Design review of the part built by this model. Coordinates are the model's own, in mm. Give positions to 0.01 mm unless a question says otherwise; leave off trailing zeros. Order: outer loops, then holes, each group sorted by start corner. A loop starts at its lowest first (then second) coordinate and runs counter-clockwise, first axis right, second up. Notation, with made-up numbers: M 74.5,-33.75 L 95.5,-33.75 A34 ccw 95.5,-2.75 Z; hole C 84,-2 d7. An arc over 180 degrees is marked long. Answer as a JSON object with one key per item and string values.
from build123d import *

# Parameters (mm, degrees)
BOSS_EXTRUDE1_DEPTH = 120
SHELL4_START        = 3
SHELL4_DEPTH        = 114
SKETCH12_W          = 3.498967662
SKETCH12_H          = 114
CUT_EXTRUDE5_DEPTH  = 2
SKETCH9_R           = 1.004458273
BOSS_EXTRUDE5_DEPTH = 10
CUT_EXTRUDE6_DEPTH  = 10
SKETCH14_W          = 1
SKETCH14_H          = 12.98385937
SKETCH14_H_2        = 14.006550136
BOSS_EXTRUDE6_DEPTH = 20


# Read off the part's stored shape, not the designer's step: Shell4
with BuildPart() as part:
    # Sketch1 → Boss-Extrude1 (new body)
    with BuildSketch(Plane(origin=(0, 0, 0), x_dir=(1, 0, 0), z_dir=(0, 1, 0))):
        with BuildLine():
            Line((-74.162924852, 98.042139327), (-73.832168128, 178.220414973))
            Line((-73.832168128, 178.220414973), (-68.833436902, 178.220414973))
            Line((-68.833436902, 178.220414973), (-68.833436902, 98.042139327))
            add(Edge.make_bspline(
                [(-68.833436902, 98.042139327), (-69.18939253, 31.860054141), (-32.378727908, -28.786275828)],
                knots=[0, 0, 0, 1, 1, 1], degree=2))
            Line((-32.378727908, -28.786275828), (-35.878727908, -35.78423441))
            add(Edge.make_bspline(
                [(-74.162924852, 98.042139327), (-75.763847477, 27.752135338), (-35.878727908, -35.78423441)],
                knots=[0, 0, 0, 1, 1, 1], degree=2))
        make_face()
    extrude(amount=BOSS_EXTRUDE1_DEPTH)

    # Shell4 outline → Shell4 (cut)
    with BuildSketch(Plane(origin=(0, 0, 0), x_dir=(1, 0, 0), z_dir=(0, 1, 0)).offset(SHELL4_START)):
        with BuildLine():
            Line((-70.8445184, 175.220414973), (-71.163065765, 98.001792885))
            add(Edge.make_bspline(
                [(-71.163065765, 98.001792885), (-71.16307999, 98.001168327), (-71.163094215, 98.000543769), (-71.16310844, 97.999919211), (-71.163122665, 97.999294653), (-71.16313689, 97.998670095), (-71.163151114, 97.998045537), (-71.163165339, 97.997420979), (-71.163179564, 97.996796421), (-71.163193789, 97.996171862), (-71.163208014, 97.995547304), (-71.163222239, 97.994922746), (-71.163236464, 97.994298188), (-71.163250689, 97.99367363), (-71.163293111, 97.991811054), (-71.163321308, 97.990573036), (-71.163349505, 97.989335018), (-71.163377702, 97.988097001), (-71.163405899, 97.986858982), (-71.163434097, 97.985620965), (-71.163462293, 97.984382945), (-71.163490491, 97.98314493), (-71.163518687, 97.98190691), (-71.163546885, 97.980668893), (-71.163575081, 97.979430874), (-71.163603278, 97.978192857), (-71.163631475, 97.976954838), (-71.163673771, 97.975097811), (-71.16368819, 97.974464701), (-71.163699727, 97.973958392), (-71.163723187, 97.972927066), (-71.163717996, 97.973159219), (-71.163755945, 97.971484687), (-71.163749131, 97.971794066), (-71.163775505, 97.970626161), (-71.163784451, 97.97023953), (-71.163799423, 97.969578445), (-71.163813375, 97.968966514), (-71.163827192, 97.968358956), (-71.163841117, 97.967746949), (-71.163868925, 97.96652446), (-71.163882828, 97.965913216), (-71.163896729, 97.965301972), (-71.163910628, 97.964690728), (-71.163924525, 97.964079485), (-71.163938422, 97.963468242), (-71.163952315, 97.962856999), (-71.163966208, 97.962245757), (-71.163980098, 97.961634515), (-71.163993987, 97.961023273), (-71.164007875, 97.960412031), (-71.16402176, 97.95980079), (-71.164035644, 97.959189549), (-71.164105055, 97.956133346), (-71.164160555, 97.953688388), (-71.16421603, 97.951243436), (-71.164271474, 97.948798484), (-71.164326897, 97.946353546), (-71.164382282, 97.943908598), (-71.164437654, 97.941463673), (-71.164492984, 97.939018734), (-71.164548299, 97.936573815), (-71.164603577, 97.93412889), (-71.164658834, 97.931683976), (-71.16471406, 97.929239064), (-71.16476926, 97.926794157), (-71.164934778, 97.919459451), (-71.165045014, 97.914569665), (-71.165155139, 97.909679898), (-71.165265157, 97.904790149), (-71.165375062, 97.899900419), (-71.165484862, 97.895010708), (-71.165594548, 97.890121015), (-71.165704128, 97.885231341), (-71.165813596, 97.880341685), (-71.165922956, 97.875452049), (-71.166032206, 97.87056243), (-71.166141347, 97.86567283), (-71.166250378, 97.860783249), (-71.166577142, 97.846114561), (-71.166794547, 97.83633551), (-71.167011514, 97.826556534), (-71.167228044, 97.816777632), (-71.167444133, 97.806998804), (-71.167659788, 97.797220051), (-71.167875001, 97.787441372), (-71.16808978, 97.777662768), (-71.168304117, 97.767884237), (-71.168518019, 97.758105782), (-71.168731482, 97.7483274), (-71.168944507, 97.738549093), (-71.169157093, 97.72877086), (-71.170217838, 97.679880069), (-71.171059425, 97.640768626), (-71.171894004, 97.601658372), (-71.172721576, 97.56254931), (-71.173542137, 97.523441433), (-71.174355694, 97.484334754), (-71.175162237, 97.445229255), (-71.175961779, 97.406124956), (-71.176754307, 97.367021836), (-71.177539831, 97.327919914), (-71.178318344, 97.288819177), (-71.179089851, 97.249719631), (-71.179854349, 97.210621274), (-71.183641802, 97.015135438), (-71.186559636, 96.858765798), (-71.189365345, 96.702415187), (-71.192058927, 96.546083598), (-71.194640389, 96.389771034), (-71.197109723, 96.233477481), (-71.199466944, 96.077202952), (-71.201712036, 95.920947426), (-71.203845018, 95.764710916), (-71.205865876, 95.608493406), (-71.207774621, 95.452294903), (-71.20957125, 95.296115396), (-71.211255765, 95.139954887), (-71.215972974, 94.671530339), (-71.21866933, 94.359323281), (-71.220917246, 94.047192171), (-71.222716731, 93.735136985), (-71.224067792, 93.423157694), (-71.224970441, 93.111254278), (-71.225424682, 92.799426705), (-71.22543053, 92.487674957), (-71.224987988, 92.175999001), (-71.224097069, 91.864398817), (-71.222757779, 91.552874376), (-71.220970129, 91.241425656), (-71.218734126, 90.930052628), (-71.210681088, 89.996160551), (-71.203519041, 89.373868515), (-71.194563692, 88.751878946), (-71.183815094, 88.130191631), (-71.171273301, 87.508806354), (-71.156938367, 86.887722903), (-71.140810347, 86.266941062), (-71.122889291, 85.646460617), (-71.103175256, 85.026281355), (-71.081668294, 84.406403059), (-71.058368459, 83.786825518), (-71.033275804, 83.167548515), (-71.006390383, 82.548571838), (-70.920355984, 80.692542137), (-70.855828771, 79.456389412), (-70.784130946, 78.221435319), (-70.70526281, 76.987678074), (-70.619224622, 75.75511588), (-70.52601661, 74.52374694), (-70.425638953, 73.293569436), (-70.318091806, 72.064581558), (-70.20337527, 70.836781468), (-70.081489423, 69.610167339), (-69.952434295, 68.384737319), (-69.816209883, 67.16048956), (-69.672816143, 65.937422197), (-69.221126701, 62.271755688), (-68.891322913, 59.832692682), (-68.532840831, 57.398329004), (-68.145679077, 54.968649529), (-67.729835685, 52.543639338), (-67.285308121, 50.123283736), (-66.812093252, 47.707568223), (-66.310187385, 45.296478532), (-65.779586225, 42.890000586), (-65.220284915, 40.488120539), (-64.632278003, 38.090824743), (-64.015559465, 35.698099773), (-63.370122691, 33.309932408), (-61.444530757, 26.501652756), (-60.094120868, 22.092657129), (-58.644686559, 17.699242409), (-57.096177659, 13.321333259), (-55.448539032, 8.958860031), (-53.701711499, 4.611759301), (-51.855632693, 0.279974273), (-49.910237914, -4.036544954), (-47.865460912, -8.33784126), (-45.721234657, -12.6239505), (-43.477492061, -16.894901644), (-41.134166666, -21.150717052), (-38.691193295, -25.391412877), (-36.148508666, -29.616999611)],
                knots=[-0.000198917, -0.000198917, -0.000198917, -0.000198917, -0.000198917, -0.000198917, -0.000198917, -0.000198917, -0.000198917, -0.000198917, -0.000198917, -0.000198917, -0.000198917, -0.000198917, -0.000198917, -0.000136719, -0.000136719, -0.000136719, -0.000136719, -0.000136719, -0.000136719, -0.000136719, -0.000136719, -0.000136719, -0.000136719, -0.000136719, -0.000136719, -0.000136719, -1.3428e-05, -1.3428e-05, -1.3428e-05, -1.3428e-05, -1.3428e-05, -1.3428e-05, -1.3428e-05, -1.3428e-05, -1.3428e-05, -1.3428e-05, -1.3428e-05, -1.3428e-05, -1.3428e-05, 4.8218e-05, 4.8218e-05, 4.8218e-05, 4.8218e-05, 4.8218e-05, 4.8218e-05, 4.8218e-05, 4.8218e-05, 4.8218e-05, 4.8218e-05, 4.8218e-05, 4.8218e-05, 4.8218e-05, 0.000109863, 0.000109863, 0.000109863, 0.000109863, 0.000109863, 0.000109863, 0.000109863, 0.000109863, 0.000109863, 0.000109863, 0.000109863, 0.000109863, 0.000109863, 0.000356445, 0.000356445, 0.000356445, 0.000356445, 0.000356445, 0.000356445, 0.000356445, 0.000356445, 0.000356445, 0.000356445, 0.000356445, 0.000356445, 0.000356445, 0.000849609, 0.000849609, 0.000849609, 0.000849609, 0.000849609, 0.000849609, 0.000849609, 0.000849609, 0.000849609, 0.000849609, 0.000849609, 0.000849609, 0.000849609, 0.001835937, 0.001835937, 0.001835937, 0.001835937, 0.001835937, 0.001835937, 0.001835937, 0.001835937, 0.001835937, 0.001835937, 0.001835937, 0.001835937, 0.001835937, 0.00578125, 0.00578125, 0.00578125, 0.00578125, 0.00578125, 0.00578125, 0.00578125, 0.00578125, 0.00578125, 0.00578125, 0.00578125, 0.00578125, 0.00578125, 0.0215625, 0.0215625, 0.0215625, 0.0215625, 0.0215625, 0.0215625, 0.0215625, 0.0215625, 0.0215625, 0.0215625, 0.0215625, 0.0215625, 0.0215625, 0.053125, 0.053125, 0.053125, 0.053125, 0.053125, 0.053125, 0.053125, 0.053125, 0.053125, 0.053125, 0.053125, 0.053125, 0.053125, 0.11625, 0.11625, 0.11625, 0.11625, 0.11625, 0.11625, 0.11625, 0.11625, 0.11625, 0.11625, 0.11625, 0.11625, 0.11625, 0.2425, 0.2425, 0.2425, 0.2425, 0.2425, 0.2425, 0.2425, 0.2425, 0.2425, 0.2425, 0.2425, 0.2425, 0.2425, 0.495, 0.495, 0.495, 0.495, 0.495, 0.495, 0.495, 0.495, 0.495, 0.495, 0.495, 0.495, 0.495, 0.963709177, 0.963709177, 0.963709177, 0.963709177, 0.963709177, 0.963709177, 0.963709177, 0.963709177, 0.963709177, 0.963709177, 0.963709177, 0.963709177, 0.963709177, 0.963709177, 0.963709177], degree=14))
            Line((-36.148508666, -29.616999611), (-34.206134458, -25.733384151))
            add(Edge.make_bspline(
                [(-34.206134458, -25.733384151), (-69.180443526, 33.523923752), (-68.833436902, 98.042139327)],
                knots=[0.025140786, 0.025140786, 0.025140786, 1, 1, 1], degree=2))
            Line((-68.833436902, 98.042139327), (-68.833436902, 175.220414973))
            Line((-68.833436902, 175.220414973), (-70.8445184, 175.220414973))
        make_face()
    extrude(amount=SHELL4_DEPTH, mode=Mode.SUBTRACT)

    # Sketch12 → Cut-Extrude5 (cut)
    with BuildSketch(Plane(origin=(-68.833436902, 0, 0), x_dir=(0, 0, -1), z_dir=(1, 0, 0))):
        with Locations((176.969898804, 60)):
            Rectangle(SKETCH12_W, SKETCH12_H)
    extrude(amount=-CUT_EXTRUDE5_DEPTH, mode=Mode.SUBTRACT)

    # Sketch9 → Boss-Extrude5 (add)
    with BuildSketch(Plane(origin=(-71.566131341, 0, -0.295229336), x_dir=(0.004125231010775818, 0, -0.9999914911983541), z_dir=(0.999991491198354, 0, 0.004125231010775817))):
        with Locations((172.925450661, 60)):
            Circle(SKETCH9_R)
    extrude(amount=BOSS_EXTRUDE5_DEPTH)

    # Sketch13 → Cut-Extrude6 (cut)
    with BuildSketch(Plane(origin=(-68.833436902, 0, 0), x_dir=(0, 0, -1), z_dir=(1, 0, 0))):
        Polygon((178.220414973, 120), (175.719029806, 120), (175.719029806, 0), (178.721352067, 0), (178.721352067, 120), align=None)
    extrude(amount=-CUT_EXTRUDE6_DEPTH, mode=Mode.SUBTRACT)

    # Sketch14 → Boss-Extrude6 (add)
    with BuildSketch(Plane(origin=(-71.566131341, 0, -0.295229336), x_dir=(0.004125231010775816, 0, -0.9999914911983541), z_dir=(0.999991491198354, 0, 0.004125231010775815))):
        with Locations((149.920607502, 15.084769689)):
            Rectangle(SKETCH14_W, SKETCH14_H)
        with Locations((149.920607502, 104.418723374)):
            Rectangle(SKETCH14_W, SKETCH14_H_2)
    extrude(amount=BOSS_EXTRUDE6_DEPTH)


solid = part.part
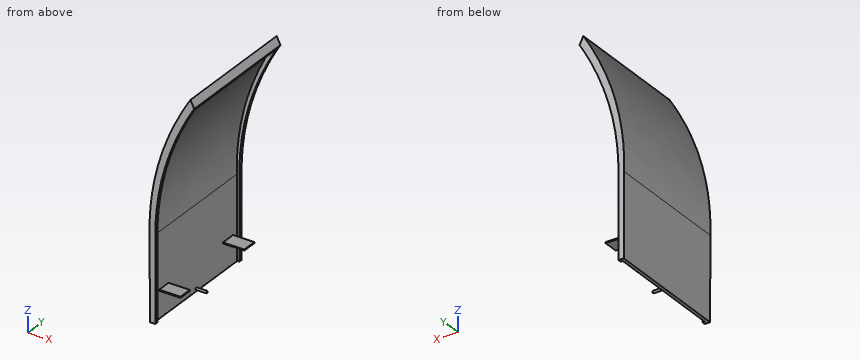
(1) We need section A-A (z = -125). Write out the cut boundary in (x, y).
Checked values:
{"outline": "M -74.05,0 L -68.83,0 L -68.83,3 L -71.05,3 L -71.05,117 L -68.83,117 L -68.83,120 L -74.05,120 Z"}
(2) We need section B-B (x = -64). Count the separate pieces of the cut face and the enclosed holes in it, plus the area to 3 significant figures.
Checked values:
{"separate pieces": "4", "enclosed holes": "0", "area": "1,430 mm^2"}
(3) To check wall thickness, follow L1, parallel to Y at x = -39.5, z = 22; L2, parallel to X at y = 32, z = 26; L3, parallel to X at y = 43.5, z = -91. State the ranges of each line that lie inside material, in increasing order. Write a range as from..to.
Checked values:
{"L1": "y = 0..3, 117..120", "L2": "x = -41.75..-38.29, -34.34..-34.05", "L3": "x = -74.22..-71.22"}
(4) Insertion check: pin 1 (12 mm diameter, centred on x = -56.5, y = 19.5, fed in from +Z); pin 2 (1.5 mm diameter, centred on y = 26, z = -58, fed in from -X); pin 3 (0.5 mm diameter, centred on x = -56, z = -150, fed in from +Y); pin 4 (18.5 mm diameter, centred on x = -52, z = -74.5, fed in from -Y). Each pin has a flat end and moves straight along its axis. Give the tip position at first contact, or say it passes through.
Checked values:
{"pin 1": "stops at z = 9.43", "pin 2": "stops at x = -71.74", "pin 3": "stops at y = 111.42", "pin 4": "passes through"}
